Input: part model. Units: mm. Frame: model coordinates. A direction names the side the tool comes from. Give positions to 0.01 mm unless a question says otherwise; leave off trailing zeros. Loops run counter-clockwise (first coordinate to the right, second up) from the corner with the lowest first, then second, coordinate; pieces in that order, holes last. Notation, with made-up numbers: M -14,15.5 L 29,15.5 A22 ccw 29,36.5 Z; hole C 13.25,84 d7. An arc over 180 degrees is marked long. Return JSON: item names as keys, results as strings. Group by question number.
```python
from build123d import *

# Parameters (mm, degrees)
F1_DEPTH = 135
F3_DEPTH = 500


with BuildPart() as f1:
    # F0 (on Front) → F1 (new body, symmetric)
    with BuildSketch(Plane.XZ):
        Polygon((464.26666, 345), (-464.26666, 345), (-322.318269, -45), (322.318269, -45), align=None)
        Polygon((290.80893, 0), (-290.80893, 0), (-400, 300), (400, 300), align=None, mode=Mode.SUBTRACT)
    extrude(amount=F1_DEPTH, both=True)

    # F2 (on Right) → F3 (cut, symmetric)
    with BuildSketch(Plane.YZ):
        Polygon((-67.5, 0), (-135, 345), (135, 345), (67.5, 0), (56.686841, -55.267259), (427.661182, -55.267259), (427.661182, 496.46467), (-274.209738, 496.46467), (-274.209738, -50), (-57.717391, -50), align=None)
    extrude(amount=F3_DEPTH, both=True, mode=Mode.SUBTRACT)


solid = f1.part
```
Item 1: Section C-C, the plane y = -5.5. Return loops of the section in (x, z), then the cut area to 3 significant figures.
Item 2: Material intervals for line 1 (Z direction, x = -91, y = 30.5); line 2 (Z direction, x = -178.5, y = 84); line 3 (X direction, y = 67, z = 206), sorted ascending. Write a range as from..to.
Item 3: First-contact query: pin 1 Ø12 at (y, z) = (-28.5, 273.5) entering from +X; pin 2 Ø4 at (y, z) = (94, 231) entering from -X; pin 3 Ø1.5 at (y, z) = (-61, 148.5) entering from +X. Flat tips, straight axial feed; report the tip coordinate or a pass-through.
Item 4: Reachability of faces 5 (the face through (346.17, -1.77, 152.1)), 6 (the face through (408.07, -1.89, 190.6)) from +Z, -Z, +X, -X, +Y, -Y: full face, straight path, thin tool, end or side. Return the list, or none.
Item 5: Section A-A, the plane x = 199. Return loops of the section in (y, z), then the cut area to 3 significant figures.
Item 6: Section D-D, the plane y = 108. Return loops of the section in (x, z).
Item 7: Section B-B, the plane z = 200. Return loops of the section in (x, y).
Item 8: Pull-direction query (X, two-part tool) for faces 1 (the face through (-5, -1, -45)), 2 (the face through (4, -1, 0)), 3 (the face through (-344.64, -1.77, 147.9)), 4 (the face through (-410.058, -1.89, 196.063)); classes: pulls with the +X half, pulls with the -X half, needs draft (parallel to the pull), parting line crosses it, or undercut.
Answer below:
{
 "1": {"outline": "M -464.27,345 L -322.32,-45 L 322.32,-45 L 464.27,345 Z; hole M -400,300 L -290.81,0 L 290.81,0 L 400,300 Z", "area": "99,500 mm^2"},
 "2": {"line 1": "-45..0, 300..345", "line 2": "300..345", "line 3": "-413.67..-365.79, 365.79..413.67"},
 "3": {"pin 1": "x = 440.43", "pin 2": "x = -423.5", "pin 3": "x = 393.02"},
 "4": {"face 5": "+Y, -Y", "face 6": "-Z, +X, +Y, -Y"},
 "5": {"outline": "M -135,345 L -126.2,300 L 126.2,300 L 135,345 Z; M -67.5,0 L -58.7,-45 L 58.7,-45 L 67.5,0 Z", "area": "17,400 mm^2"},
 "6": {"outline": "M -464.27,345 L -414.04,207 L -366.15,207 L -400,300 L 400,300 L 366.15,207 L 414.04,207 L 464.27,345 Z"},
 "7": {"outline": "M -411.49,-106.63 L -363.6,-106.63 L -363.6,106.63 L -411.49,106.63 Z; M 363.6,-106.63 L 411.49,-106.63 L 411.49,106.63 L 363.6,106.63 Z"},
 "8": {"face 1": "needs draft", "face 2": "undercut", "face 3": "undercut", "face 4": "pulls with the -X half"}
}
